Could you check a few things on this model? Use its own coordinates, in mm. Face numbers are marked on the shaded views. A direction names the side the tool comes from. Round coordinates to 2 decimals unless told otherwise and drop trailing zeros. Write each loop counter-clockwise with the first axis right and the second up, starting at its lowest first coordinate (ties: lowest second). Pieces come first, ordered by that corner, then holes. Notation, with made-up numbers: M -25,89 L -11,89 A21 ccw -11,93 Z; hole C -40,44 d1. An arc over 180 degrees is marked long. One line per question, with ' | ' between items. Start each with the question number.
```python
from build123d import *

# Parameters (mm, degrees)
BOSS_EXTRUDE1_DEPTH      = 20
BOSS_EXTRUDE1_DEPTH_BACK = 20
SKETCH1_R                = 30
SKETCH1_R_2              = 21
BOSS_EXTRUDE2_DEPTH      = 20
BOSS_EXTRUDE2_DEPTH_BACK = 20
SKETCH2_R                = 100
SKETCH2_R_2              = 21
CUT_EXTRUDE1_DEPTH       = 20
CUT_EXTRUDE1_DEPTH_BACK  = 20


with BuildPart() as part:
    # Sketch1 → Boss-Extrude1 (new, two sides: drawn at the far end of the back side and taken through both)
    with BuildSketch(Plane.XY.offset(-BOSS_EXTRUDE1_DEPTH_BACK)):
        Circle(SKETCH1_R)
        Circle(SKETCH1_R_2, mode=Mode.SUBTRACT)
    extrude(amount=BOSS_EXTRUDE1_DEPTH + BOSS_EXTRUDE1_DEPTH_BACK)

    # Sketch2 → Boss-Extrude2 (add, two sides: drawn at the far end of the back side and taken through both)
    with BuildSketch(Plane.XY.offset(-BOSS_EXTRUDE2_DEPTH_BACK)):
        Circle(SKETCH2_R)
        Circle(SKETCH2_R_2, mode=Mode.SUBTRACT)
    extrude(amount=BOSS_EXTRUDE2_DEPTH + BOSS_EXTRUDE2_DEPTH_BACK)

    # Sketch3 → Cut-Extrude1 (cut, two sides: drawn at the far end of the back side and taken through both)
    with BuildSketch(Plane.XY.offset(-CUT_EXTRUDE1_DEPTH_BACK)):
        with BuildLine():
            Line((-27.041634566, 46.837484988), (-34.641016151, 60))
            ThreePointArc((-34.641016151, 60), (-35.429873939, 68.273268354), (-29.692299558, 74.285714286))
            ThreePointArc((-29.692299558, 74.285714286), (0, 80), (29.692299558, 74.285714286))
            ThreePointArc((29.692299558, 74.285714286), (35.429873939, 68.273268354), (34.641016151, 60))
            Line((34.641016151, 60), (27.041634566, 46.837484988))
            ThreePointArc((27.041634566, 46.837484988), (21.840560017, 42.45483732), (15.039311341, 42.412487717))
            ThreePointArc((15.039311341, 42.412487717), (0, 45), (-15.039311341, 42.412487717))
            ThreePointArc((-15.039311341, 42.412487717), (-21.840560017, 42.45483732), (-27.041634566, 46.837484988))
        make_face()
        with BuildLine():
            Line((46.837484988, 27.041634566), (60, 34.641016151))
            ThreePointArc((60, 34.641016151), (68.273268354, 35.429873939), (74.285714286, 29.692299558))
            ThreePointArc((74.285714286, 29.692299558), (80, 0), (74.285714286, -29.692299558))
            ThreePointArc((74.285714286, -29.692299558), (68.273268354, -35.429873939), (60, -34.641016151))
            Line((60, -34.641016151), (46.837484988, -27.041634566))
            ThreePointArc((46.837484988, -27.041634566), (42.45483732, -21.840560017), (42.412487717, -15.039311341))
            ThreePointArc((42.412487717, -15.039311341), (45, 0), (42.412487717, 15.039311341))
            ThreePointArc((42.412487717, 15.039311341), (42.45483732, 21.840560017), (46.837484988, 27.041634566))
        make_face()
        with BuildLine():
            Line((27.041634566, -46.837484988), (34.641016151, -60))
            ThreePointArc((34.641016151, -60), (35.429873939, -68.273268354), (29.692299558, -74.285714286))
            ThreePointArc((29.692299558, -74.285714286), (0, -80), (-29.692299558, -74.285714286))
            ThreePointArc((-29.692299558, -74.285714286), (-35.429873939, -68.273268354), (-34.641016151, -60))
            Line((-34.641016151, -60), (-27.041634566, -46.837484988))
            ThreePointArc((-27.041634566, -46.837484988), (-21.840560017, -42.45483732), (-15.039311341, -42.412487717))
            ThreePointArc((-15.039311341, -42.412487717), (0, -45), (15.039311341, -42.412487717))
            ThreePointArc((15.039311341, -42.412487717), (21.840560017, -42.45483732), (27.041634566, -46.837484988))
        make_face()
        with BuildLine():
            Line((-46.837484988, -27.041634566), (-60, -34.641016151))
            ThreePointArc((-60, -34.641016151), (-68.273268354, -35.429873939), (-74.285714286, -29.692299558))
            ThreePointArc((-74.285714286, -29.692299558), (-80, 0), (-74.285714286, 29.692299558))
            ThreePointArc((-74.285714286, 29.692299558), (-68.273268354, 35.429873939), (-60, 34.641016151))
            Line((-60, 34.641016151), (-46.837484988, 27.041634566))
            ThreePointArc((-46.837484988, 27.041634566), (-42.45483732, 21.840560017), (-42.412487717, 15.039311341))
            ThreePointArc((-42.412487717, 15.039311341), (-45, 0), (-42.412487717, -15.039311341))
            ThreePointArc((-42.412487717, -15.039311341), (-42.45483732, -21.840560017), (-46.837484988, -27.041634566))
        make_face()
    extrude(amount=CUT_EXTRUDE1_DEPTH + CUT_EXTRUDE1_DEPTH_BACK, mode=Mode.SUBTRACT)


solid = part.part
```
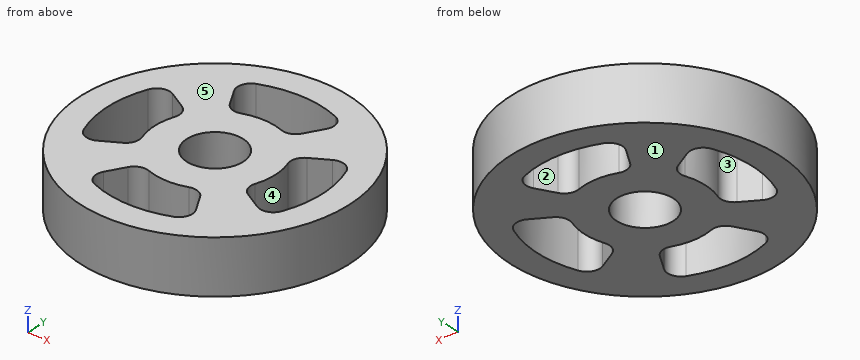
1. If we mould it in two halves opening along X, with no side actions, what happens to the marked faces 3, 4 and 5? For each: released by +X, released by -X, zero draft, split by the parting line, or undercut.
2. Which directions (+Z, -Z, +X, -X, +Y, -Y) give clear straight access to the entire face, cutting with the end or side of a thin tool? Please do the marked faces 1 and 2.
3. Suppose I cut it at D-D (x = 64). Write out the boundary of the cut face in (y, z), and give its area (3 significant figures).
4. Suppose I cut it at A-A (x = 0). Write out the boundary of the cut face in (y, z), and give its area (3 significant figures).
5. I'm going to push flat-ended pins straight in: P1, Ø5, axis at y = -13.5, z = 9.5, coming from the -X side; P2, Ø1.5, axis at y = 12.5, z = 5, coming from the -X side; P3, Ø8, axis at y = -24, z = -1, coming from the -X side. Where does each tip first touch, or does it pass through?
6. I need wall thicknesses on line 1 along X through (y, z) = (-11, 4); line 2 along Y through (x, z) = (16, 17); line 3 along X through (y, z) = (-27, 16.5). Which ranges of each line are inside material? Lowest first, please. Write a range as from..to.
7. Suppose I cut it at C-C (z = -7.5). Count the separate pieces of the cut face and the enclosed holes in it, and give its area (3 significant figures).
Computed:
1) face 3: undercut | face 4: undercut | face 5: zero draft
2) face 1: -Z, +X, -X, +Y, -Y | face 2: +Z, -Z
3) outline: M -76.84,-20 L -35.93,-20 L -35.93,20 L -76.84,20 Z; M 35.93,-20 L 76.84,-20 L 76.84,20 L 35.93,20 Z | area: 3,270 mm²
4) outline: M -100,-20 L -80,-20 L -80,20 L -100,20 Z; M -45,-20 L -21,-20 L -21,20 L -45,20 Z; M 21,-20 L 45,-20 L 45,20 L 21,20 Z; M 80,-20 L 100,-20 L 100,20 L 80,20 Z | area: 3,520 mm²
5) P1: stops at x = -99.39 | P2: stops at x = -99.31 | P3: stops at x = -97.98
6) line 1: x = -99.39..-79.24, -43.63..-17.89, 17.89..43.63, 79.24..99.39 | line 2: y = -98.71..-78.38, -42.13..-13.6, 13.6..42.13, 78.38..98.71 | line 3: x = -96.29..-75.31, -46.77..46.77, 75.31..96.29
7) separate pieces: 1 | enclosed holes: 5 | area: 21,200 mm²
